Print and shaded views of the part. All mm, measured from the part's lowest x, y and z. A direction names the side the tool comes from. Coordinates: 2 decimals unless noted, no trailing zeros. Order: outer loops, then holes, each group sorted by start corner. A loop starts at its lowest first (then second) coordinate and runs counter-clockwise, first axis right, second up. Notation, with made-up numbers: (10.5, 29.5) -> (33.5, 29.5) arc R34 ccw to (33.5, 67.5) -> close; hole circle Ø11 at (-10.75, 77). An arc over 180 degrees is marked (long way). Return JSON: item names as keys, results as strings. Group by question number.
1) Pull direction X, two halves, no side cores. Call the marked faces 3, 4 and 5: +X half, -X half, draft (parallel to the pull), parting line (faces both ways), or undercut.
2) Cut at D-D (z = 19.5). Write the cut outline in (x, y), and give its area (3 significant figures).
3) Cut at A-A (x = 24.5). Write the cut outline in (y, z).
4) Cut at B-B (z = 35). Write the cut outline in (x, y).
5) Flat gauge pins, fed straight in: pin 1 (22.5 mm diameter, centred on x = 24.5, z = 35, fed in from +Y); pin 2 (3.5 mm diameter, centred on x = 40, z = 19.5, fed in from -Y). Where does each tip first touch, or does it go through?
6) Probe line 1 (X direction, y = 67.25, z = 19.5); line 2 (Z direction, x = 24, y = 60); line 3 (X direction, y = 25, z = 41). List the from-to ranges inside material, lowest first.
7) Cut at C-C (y = 23.5). Write the cut outline in (x, z), and give its area (3 significant figures).
8) Which spindle directions (+Z, -Z, +X, -X, +Y, -Y) get a long thin tool onto all of the face, cutting with end or side? Do the marked faces 1 and 2. Say none if no direction does.
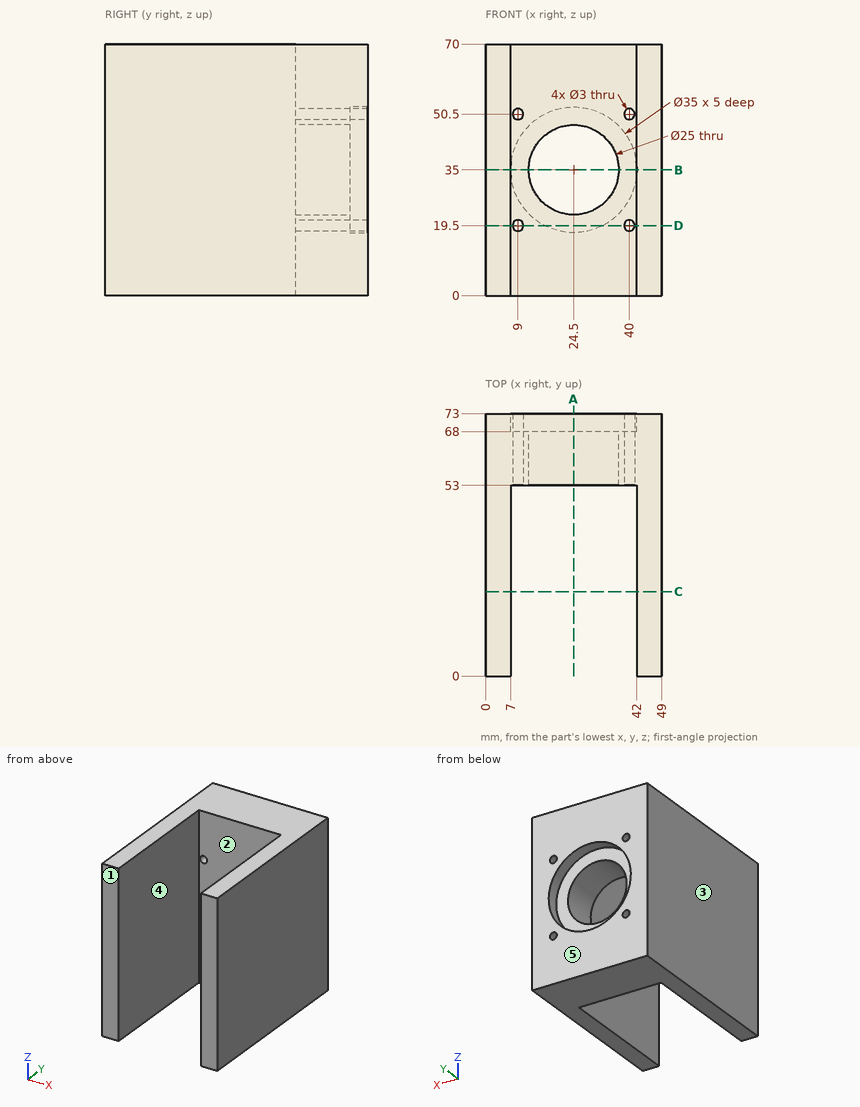
Answers below:
{
 "1": {"face 3": "-X half", "face 4": "undercut", "face 5": "draft"},
 "2": {"outline": "(0, 0) -> (7, 0) -> (7, 53) -> (7.5, 53) -> (7.5, 73) -> (0, 73) -> close; (10.5, 53) -> (38.5, 53) -> (38.5, 73) -> (32.62, 73) -> (32.62, 68) -> (16.38, 68) -> (16.38, 73) -> (10.5, 73) -> close; (41.5, 53) -> (42, 53) -> (42, 0) -> (49, 0) -> (49, 73) -> (41.5, 73) -> close", "area": "1,520 mm^2"},
 "3": {"outline": "(53, 0) -> (73, 0) -> (73, 17.5) -> (68, 17.5) -> (68, 22.5) -> (53, 22.5) -> close; (53, 47.5) -> (68, 47.5) -> (68, 52.5) -> (73, 52.5) -> (73, 70) -> (53, 70) -> close"},
 "4": {"outline": "(0, 0) -> (7, 0) -> (7, 53) -> (12, 53) -> (12, 68) -> (7, 68) -> (7, 73) -> (0, 73) -> close; (37, 53) -> (42, 53) -> (42, 0) -> (49, 0) -> (49, 73) -> (42, 73) -> (42, 68) -> (37, 68) -> close"},
 "5": {"pin 1": "passes through", "pin 2": "stops at y = 53"},
 "6": {"line 1": "x = 0 to 7.5, 10.5 to 38.5, 41.5 to 49", "line 2": "z = 0 to 22.51, 47.49 to 70", "line 3": "x = 0 to 7, 42 to 49"},
 "7": {"outline": "(0, 0) -> (7, 0) -> (7, 70) -> (0, 70) -> close; (42, 0) -> (49, 0) -> (49, 70) -> (42, 70) -> close", "area": "980 mm^2"},
 "8": {"face 1": "+Z, -Z, +X, -X, -Y", "face 2": "+Z, -Z, -Y"}
}
